Autodesk Inventor part; units mm, degrees
ref_plane "YZ Plane" through (0, 0, 0) normal (1, 0, 0) x (0, 1, 0)
ref_plane "XZ Plane" through (0, 0, 0) normal (0, 1, 0) x (-1, 0, 0)
ref_plane "XY Plane" through (0, 0, 0) normal (0, 0, 1) x (1, 0, 0)
sketch "スケッチ1" plane through (0, 0, 0) normal (0, 0, 1) x (1, 0, 0)
  line L0 (0, 0) -> (370, 0)
  line L1 (370, 0) -> (370, 250)
  line L2 (370, 250) -> (320, 250)
  line L3 (320, 250) -> (320, 240)
  line L4 (320, 240) -> (50, 240)
  line L5 (50, 240) -> (50, 250)
  line L6 (50, 250) -> (0, 250)
  line L7 (0, 250) -> (0, 0)
  dimension "d0" = 50
  dimension "d1" = 10
  dimension "d2" = 250
  dimension "d3" = 370
extrude "押し出し1" add sketch "スケッチ1" along normal blind 10
chamfer "面取り1" distance 5 angle 45 3 edges at (185, 0, 10) (0, 125, 10) (370, 125, 10)
chamfer "面取り2" distance 10 angle 45 4 edges at (0, 0, 2.5) (370, 0, 2.5) (370, 250, 2.5) (0, 250, 2.5)
fillet "フィレット2" radius 5 4 edges at (30, 250, 10) (30, 250, 0) (340, 250, 10) (340, 250, 0)
sketch "スケッチ2" plane through (320, 240, 0) normal (-1, 0, 0) x (0, 0, 1)
  arc A0 (10, 5) -> (0, 5) centre (5, 5) ccw
  circle A1 centre (5, 5) radius 2
  point P0 (0, -240)
  dimension "d14" = 4
extrude "押し出し2" cut sketch "スケッチ2" along normal blind 280 and the other way blind 10
fillet "フィレット3" radius 2 2 edges at (185, 240, 10) (185, 240, 0)
sketch "スケッチ3" plane through (0, 0, 0) normal (0, 0, -1) x (-1, 0, 0)
  line L0 (-10, 0) -> (-360, 0)
  line L1 (-185, 0) -> (-185, 240) construction
  line L2 (-50, 240) -> (-320, 240)
  line L3 (-20, 20) -> (-350, 20)
  line L4 (-350, 20) -> (-350, 220)
  line L5 (-350, 220) -> (-20, 220)
  line L6 (-20, 220) -> (-20, 20)
  line L7 (-20, 20) -> (-350, 220) construction
  line L8 (-350, 20) -> (-20, 220) construction
  line L9 (-370, 10) -> (-370, 240)
  point P0 (0, 0)
  point P1 (-185, 120)
  dimension "d20" = 20
  dimension "d21" = 20
  dimension "d22" = 200
extrude "押し出し3" cut sketch "スケッチ3" against normal blind 1
properties part number "PCパーツ2"
Verification items for the finished model (mm, model axes). A direction names the side the tool comes from. Give positions to 0.01 mm unless a question says otherwise; leave off trailing zeros. Loops run counter-clockwise (first coordinate to the right, second up) from the corner with the lowest first, then second, coordinate; pieces in that order, holes last. Notation, with made-up numbers: (-25.5, 73.25) - (8.5, 73.25) arc R24 cw to (8.5, 99.25) - close; hole circle Ø2 at (25.25, 51.25). An arc over 180 degrees is marked (long way). Write item = value, one per line. Start each with the question number.
Q1. Cross-section at B-B, the plane x = 258.5. Enter the section's corners in (y, z), and give its area (3 significant figures).
Q2. Mould release check, pull along X, two halves, no side actions. Record for faces 3 (the face through (50, 242.6, 4.9)), 4 (the face through (5, 5, 4)), 5 (the face through (365, 245, 5)), 6 (the face through (182, 127, 10)): released by +X, released by -X, zero draft, split by the parting line, or undercut.
Q3. Depth check by flat-ended pin: P1, Ø5, axis at y = 242, z = 7, coming from the -X side; P2, Ø12, axis at x = 62, y = 92, coming from the -Z side; P3, Ø1.5, axis at x = 279, z = 7.5, coming from the +Y side. Enter the tip coordinate at first touch or a pass-through.
Q4. Thickness scan on line 1 (Y direction, x = 45.75, z = 5); line 2 (Z direction, x = 46, y = 245); line 3 (Z direction, x = 42, y = 201.5). Record the ranges inside material, lowest first.
Q5. Cross-section at A-A, the plane y = 127. Enter the section's corners in (x, z).
Q6. Tool access check on faces 1 (the face through (187, 121, 1)), 2 (the face through (365, 5, 4)). Record the directions out of +Z, -Z, +X, -X, +Y, -Y that give a thin tool (end or side, any length) a straight path to the whole face; none if there is none.
Answer key:
q1.outline = (0, 0) - (20, 0) - (20, 1) - (220, 1) - (220, 0) - (238, 0) arc R2 ccw to (240, 2) - (240, 8) arc R2 ccw to (238, 10) - (5, 10) - (0, 5) - close
q1.area = 2,190 mm^2
q2.face_3 = undercut
q2.face_4 = released by -X
q2.face_5 = released by +X
q2.face_6 = zero draft
q3.P1 = 0.23
q3.P2 = 1
q3.P3 = 240
q4.line_1 = 0 to 243, 247 to 250
q4.line_2 = 0 to 3, 7 to 10
q4.line_3 = 1 to 10
q5.outline = (0, 0) - (20, 0) - (20, 1) - (350, 1) - (350, 0) - (370, 0) - (370, 5) - (365, 10) - (5, 10) - (0, 5) - close
q6.face_1 = -Z
q6.face_2 = +Z, -Z, +X, -Y
